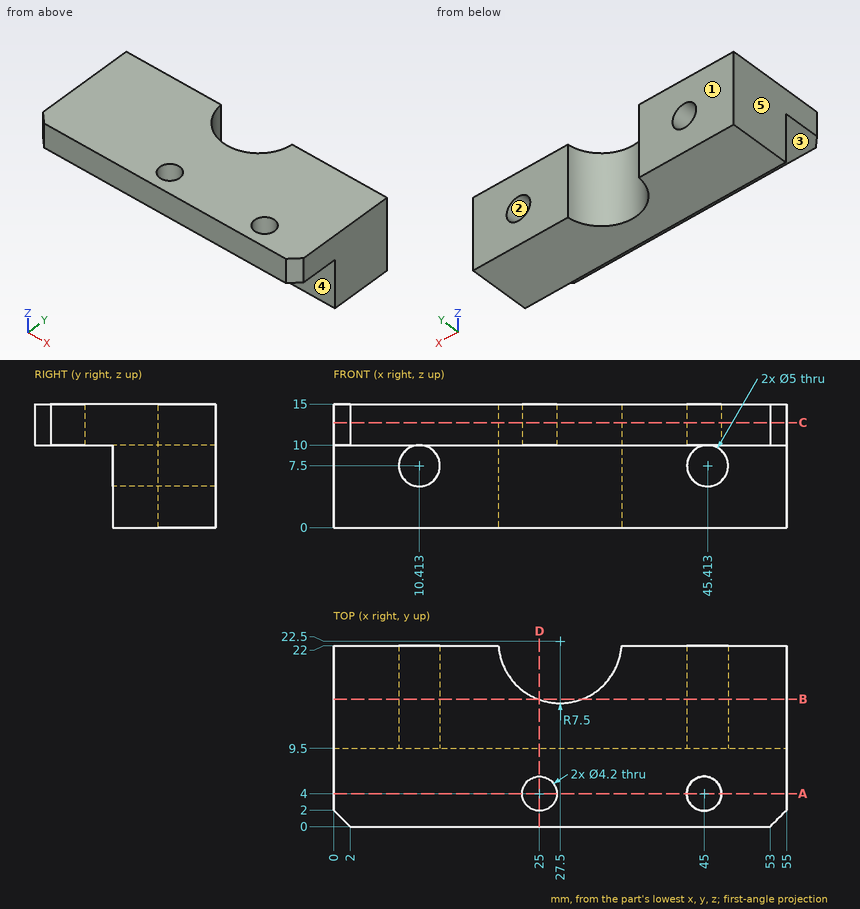
Design review of the part shown in the three views and the two pictorial views. Dimensions are in mm from the part's minimum x, y and z. A direction names the side the tool comes from. Coordinates: 2 decimals unless noted, no trailing zeros. Order: outer loops, then holes, each group sorted by start corner. A loop starts at its lowest first (then second) coordinate and runs counter-clockwise, first axis right, second up. Notation, with made-up numbers: (39.5, -30) -> (45.5, -30) arc R25 cw to (45.5, -7) -> close; hole circle Ø5 at (61, 28.25). An arc over 180 degrees is marked (long way). Use one line per item in the form item = value. Start each with the question number.
(1) For probe 1 along X at (y, z) = (12.25, 7.5); probe 2 along X at (y, z) = (16.25, 7.5) (1 decimal); probe 3 along X at (y, z) = (17, 7.5) (1 decimal), list the stretches that pass through material, from the lowest coordinate up.
(2) Insertion check: pin 1 (3 mm diameter, centred on x = 18.5, z = 2.5, fed in from -Y); pin 2 (3.5 mm diameter, centred on x = 45, y = 4, fed in from +Z); pin 3 (1 mm diameter, centred on x = 17, y = 6.5, fed in from -Z); pin 4 (8 mm diameter, centred on x = 29, z = 5, fed in from +Y). Each pin has a flat end and moves straight along its axis. Give the tip position at first contact, or say it passes through.
(3) Add section D-D on x = 25. State the section outline as (y, z) points, plus the area to 3 significant figures.
(4) Add section B-B on y = 15.5. State the section outline as (x, z) points, plus the area to 3 significant figures.
(5) Add section C-C on z = 12.75. State the section outline as (x, y) points, plus the area to 3 significant figures.
(6) Add section A-A on y = 4. State the section outline as (x, z) points, plus the area to 3 significant figures.
(7) For the marked faces 4 and 5, list the 3-axis set-ups (+Z, -Z, +X, -X, +Y, -Y) from which the entire face can be reached by the end or side of a thin tool; tool diameter is ignored.
(8) The part is to be moulded in two halves that separate along Z. For the marked faces 1, 2 and 3, say which applies: +Z half, -Z half, draft (parallel to the pull), parting line (faces both ways), or undercut.
Answer block:
q1.probe_1 = 0 to 7.91, 12.91 to 42.91, 47.91 to 55
q1.probe_2 = 0 to 7.9, 12.9 to 23.4, 31.6 to 42.9, 47.9 to 55
q1.probe_3 = 0 to 7.9, 12.9 to 22.4, 32.6 to 42.9, 47.9 to 55
q2.pin_1 = 9.5
q2.pin_2 = through
q2.pin_3 = 10
q2.pin_4 = 17.4
q3.outline = (0, 10) -> (1.9, 10) -> (1.9, 15) -> (0, 15) -> close; (6.1, 10) -> (9.5, 10) -> (9.5, 0) -> (15.43, 0) -> (15.43, 15) -> (6.1, 15) -> close
q3.area = 115 mm²
q4.outline = (0, 0) -> (24.81, 0) -> (24.81, 15) -> (0, 15) -> close; (30.19, 0) -> (55, 0) -> (55, 15) -> (30.19, 15) -> close; hole circle Ø5 at (10.41, 7.5); hole circle Ø5 at (45.41, 7.5)
q4.area = 705 mm²
q5.outline = (0, 2) -> (2, 0) -> (53, 0) -> (55, 2) -> (55, 22) -> (34.98, 22) arc R7.5 cw to (20.02, 22) -> (0, 22) -> close; hole circle Ø4.2 at (25, 4); hole circle Ø4.2 at (45, 4)
q5.area = 1,100 mm²
q6.outline = (0, 10) -> (22.9, 10) -> (22.9, 15) -> (0, 15) -> close; (27.1, 10) -> (42.9, 10) -> (42.9, 15) -> (27.1, 15) -> close; (47.1, 10) -> (55, 10) -> (55, 15) -> (47.1, 15) -> close
q6.area = 233 mm²
q7.face_4 = -Z, +X, -X, -Y
q7.face_5 = +Z, -Z, -X, +Y, -Y
q8.face_1 = draft
q8.face_2 = undercut
q8.face_3 = -Z half
